```python
from build123d import *

# Parameters (mm, degrees)
F0_W     = 25.4
F0_H     = 3.3782
F0_W_2   = 3.3782
F0_W_3   = 13.335
F0_H_2   = 21.3868
F0_H_3   = 13.335
F3_R     = 13.335
F4_DEPTH = 84.2274001
F5_R     = 13.335
F6_DEPTH = 76.2010001


with BuildPart() as f1:
    # F0 (on Top) → F1 (revolve)
    with BuildSketch(Plane.XY):
        with Locations((-29.4132, 15.0241)):
            Rectangle(F0_W, F0_H)
        with Locations((-15.0241, 15.0241)):
            Rectangle(F0_W_2, F0_H)
        with Locations((-6.6675, 15.0241)):
            Rectangle(F0_W_3, F0_H)
        Polygon((13.335, 16.7132), (0, 16.7132), (0, 13.335), (3.2870748948, 13.335), (13.335, 13.335), align=None)
        with Locations((15.0241, 15.0241)):
            Rectangle(F0_W_2, F0_H)
        with Locations((29.4132, 15.0241)):
            Rectangle(F0_W, F0_H)
    revolve(axis=Axis((-21.0566, 0, 0), (-1, 0, 0)))

    # F0 (on Top) → F2 (revolve)
    with BuildSketch(Plane.XY):
        with Locations((-15.0241, -27.4066)):
            Rectangle(F0_W_2, F0_H_2)
        with Locations((-15.0241, -15.0241)):
            Rectangle(F0_W_2, F0_H)
        with Locations((-15.0241, -6.6675)):
            Rectangle(F0_W_2, F0_H_3)
        with Locations((-15.0241, 6.6675)):
            Rectangle(F0_W_2, F0_H_3)
        with Locations((-15.0241, 15.0241)):
            Rectangle(F0_W_2, F0_H)
        with Locations((-15.0241, 27.4066)):
            Rectangle(F0_W_2, F0_H_2)
    revolve(axis=Axis((0, 19.05, 0), (0, -1, 0)))

    # F3 (on face) → F4 (cut, through all)
    with BuildSketch(Plane.YZ.offset(42.1132)):
        Circle(F3_R)
    extrude(amount=-F4_DEPTH, mode=Mode.SUBTRACT)

    # F5 (on face) → F6 (cut, through all)
    with BuildSketch(Plane(origin=(0, 38.1, 0), x_dir=(-1, 0, 0), z_dir=(0, 1, 0))):
        Circle(F5_R)
    extrude(amount=-F6_DEPTH, mode=Mode.SUBTRACT)


solid = f1.part
```
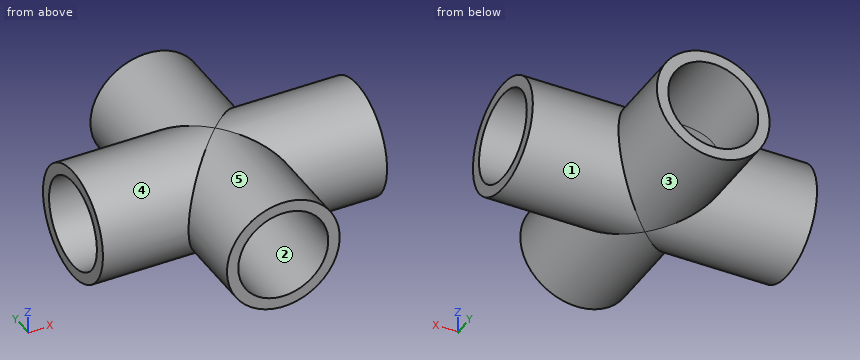
Geometry check sheet. Reference: the model listing, model coordinates, mm. Face numbers are marked on the shaded views. A direction names the side the tool comes from. Round coordinates to 2 decimals unless told otherwise and drop trailing zeros. Order: outer loops, then holes, each group sorted by start corner. A loop starts at its lowest first (then second) coordinate and runs counter-clockwise, first axis right, second up. Notation, with made-up numbers: (-34.5, 9.25) - (16.5, 9.25) arc R19 cw to (16.5, 18.25) - close; hole circle Ø2 at (47, 58.5). An arc over 180 degrees is marked (long way). Use a Markdown table: item, result. Add a question column.
(1) Sectioned sample at D-D, the plane z = 5.5. Enter the section's corners in (x, y), and give its area (3 significant figures).
(2) Tool access check on the marked faces 1, 2, 3, 4 and 5. Record the directions out of +Z, -Z, +X, -X, +Y, -Y that give a thin tool (end or side, any length) a straight path to the whole face; none if there is none.
(3) Depth check by flat-ended pin: pin 1 (5 mm diameter, centred on x = 10, y = 28.5, fed in from -Z); pin 2 (8 mm diameter, centred on x = -27.5, z = -5.5, fed in from -Y); pin 3 (8 mm diameter, centred on x = -6, y = 29.5, fed in from +Z); pin 4 (16 mm diameter, centred on x = 0, z = 0, fed in from +Y). Enter the tip coordinate at first touch or a pass-through.
(4) Sectioned sample at B-B, the plane y = 5. Enter the section's corners in (x, z) (3 decimals).
(5) Material ranges on line 1 along Y through (x, z) = (-24.5, 0) (3 decimals), recorded low to high. Write a range as [from, to].
(6) Sectioned sample at A-A, the plane z = 0. Enter the section's corners in (x, y) (3 decimals).
(7) Sectioned sample at C-C, the plane x = -33. Enter the section's corners in (y, z) (3 decimals).
Answers below:
| question | item | result |
|---|---|---|
| 1 | outline | (-42.11, -15.78) - (-15.78, -15.78) - (-15.78, -38.1) - (-12.15, -38.1) - (-12.15, -12.15) - (-42.11, -12.15) - close; (-42.11, 12.15) - (-12.15, 12.15) - (-12.15, 38.1) - (-15.78, 38.1) - (-15.78, 15.78) - (-42.11, 15.78) - close; (12.15, -38.1) - (15.78, -38.1) - (15.78, -15.78) - (42.11, -15.78) - (42.11, -12.15) - (12.15, -12.15) - close; (12.15, 12.15) - (42.11, 12.15) - (42.11, 15.78) - (15.78, 15.78) - (15.78, 38.1) - (12.15, 38.1) - close |
| 1 | area | 760 mm² |
| 2 | face 1 | +X |
| 2 | face 2 | +Y, -Y |
| 2 | face 3 | +Y |
| 2 | face 4 | -X |
| 2 | face 5 | -Y |
| 3 | pin 1 | z = -14.94 |
| 3 | pin 2 | y = -16.65 |
| 3 | pin 3 | z = 16.59 |
| 3 | pin 4 | through |
| 4 | outline | (-42.113, -15.948) - (-5, -15.948) arc R16.713 ccw to (5, -15.948) - (42.113, -15.948) - (42.113, -12.362) - (5, -12.362) arc R13.335 cw to (-5, -12.362) - (-42.113, -12.362) - close; (-42.113, 12.362) - (-5, 12.362) arc R13.335 cw to (5, 12.362) - (42.113, 12.362) - (42.113, 15.948) - (5, 15.948) arc R16.713 ccw to (-5, 15.948) - (-42.113, 15.948) - close |
| 5 | line 1 | [-16.713, -13.335], [13.335, 16.713] |
| 6 | outline | (-42.113, -16.713) - (-16.713, -16.713) - (-16.713, -38.1) - (-13.335, -38.1) - (-13.335, -13.335) - (-42.113, -13.335) - close; (-42.113, 13.335) - (-13.335, 13.335) - (-13.335, 38.1) - (-16.713, 38.1) - (-16.713, 16.713) - (-42.113, 16.713) - close; (13.335, -38.1) - (16.713, -38.1) - (16.713, -16.713) - (42.113, -16.713) - (42.113, -13.335) - (13.335, -13.335) - close; (13.335, 13.335) - (42.113, 13.335) - (42.113, 16.713) - (16.713, 16.713) - (16.713, 38.1) - (13.335, 38.1) - close |
| 7 | outline | circle Ø33.426 at (0, 0); hole circle Ø26.67 at (0, 0) |
